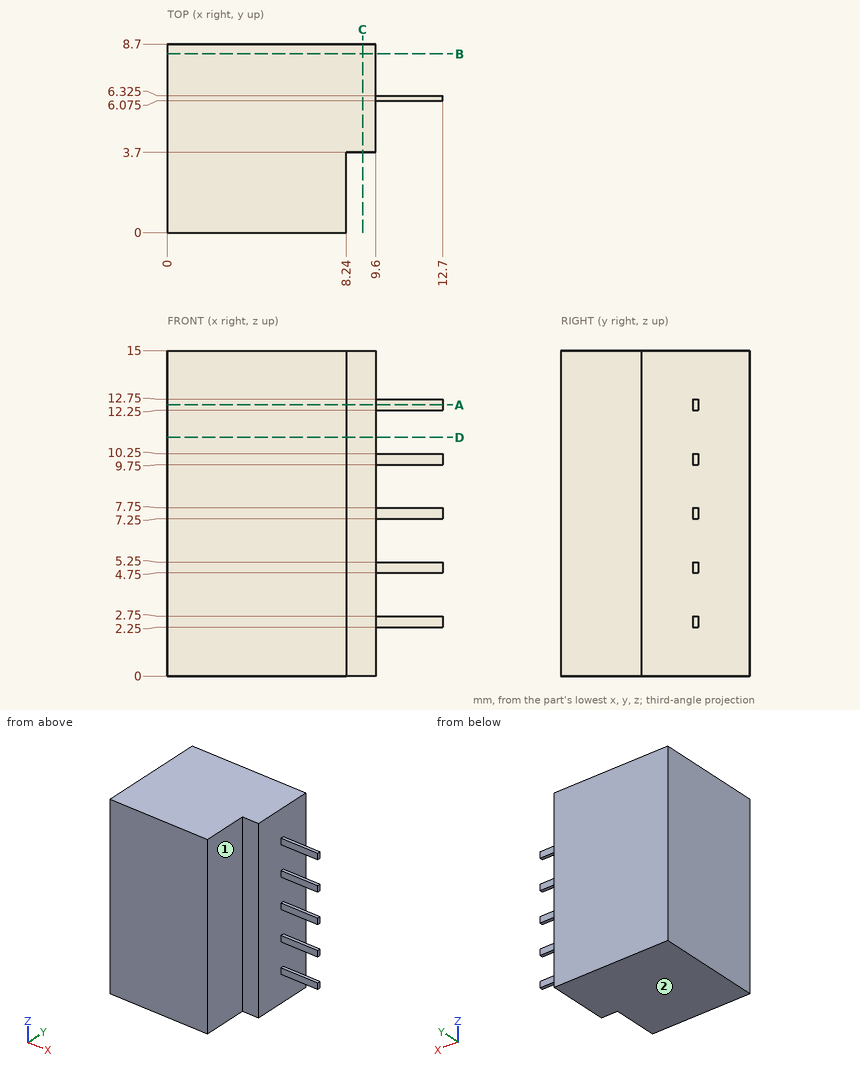
Geometry check sheet. Reference: drawing and pictorial views, mm from the part's lowest x, y, z. A direction names the side the tool comes from. Give positions to 0.01 mm unless a question says otherwise; leave off trailing zeros. Write each loop counter-clockwise with the first axis right and the second up, starting at its lowest first coordinate (ties: lowest second). Pieces come first, ordered by that corner, then holes. Notation, with made-up numbers: M 60,23.25 L 105,23.25 A25 ccw 105,55.25 Z; hole C 59.25,15 d7. An arc over 180 degrees is marked long. Use CSV: the item, a comma, the result in double quotes.
1) Cross-section at C-C (x = 9). Enter the section's corners in (y, z), plus the area to 3 significant figures.
Final values:
outline,"M 3.7,0 L 8.7,0 L 8.7,15 L 3.7,15 Z"
area,"75.0 mm²"
2) Cross-section at A-A (z = 12.5). Enter the section's corners in (x, y) (3 decimals).
Final values:
outline,"M 0,0 L 8.24,0 L 8.24,3.7 L 9.6,3.7 L 9.6,6.075 L 12.7,6.075 L 12.7,6.325 L 9.6,6.325 L 9.6,8.7 L 0,8.7 Z"
3) Cross-section at D-D (z = 11). Enter the section's corners in (x, y).
Final values:
outline,"M 0,0 L 8.24,0 L 8.24,3.7 L 9.6,3.7 L 9.6,8.7 L 0,8.7 Z"
4) Cross-section at B-B (y = 8.25). Enter the section's corners in (x, z), plus the area to 3 significant figures.
Final values:
outline,"M 0,0 L 9.6,0 L 9.6,15 L 0,15 Z"
area,"144 mm²"
5) Access from +Z, -Z, +X, -X, +Y, -Y to the whole of each face (thin tool, end or side, straight path). Record for the marked faces 1 and 2.
Final values:
face 1,"+Z, -Z, +X, -Y"
face 2,"-Z, +X, -X, +Y, -Y"
6) Material ranges on line 1 along Y through (x, z) = (11, 2.5) (3 decimals); line 2 along Y through (x, z) = (9.25, 11.5); line 3 along X through (y, z) = (5.25, 11.25), recorded low to high.
Final values:
line 1,"6.075 to 6.325"
line 2,"3.7 to 8.7"
line 3,"0 to 9.6"
7) Go/stop test with flat-tipped pins: pin 1 Ø2 at (y, z) = (3, 10.5) entering from -X; pin 2 Ø0.6 at (x, z) = (12, 7.5) entering from -Y (3 decimals); pin 3 Ø3 at (y, z) = (1, 5) entering from +X. Record where each tip stops, or that it passes through.
Final values:
pin 1,"x = 0"
pin 2,"y = 6.075"
pin 3,"x = 8.24"
